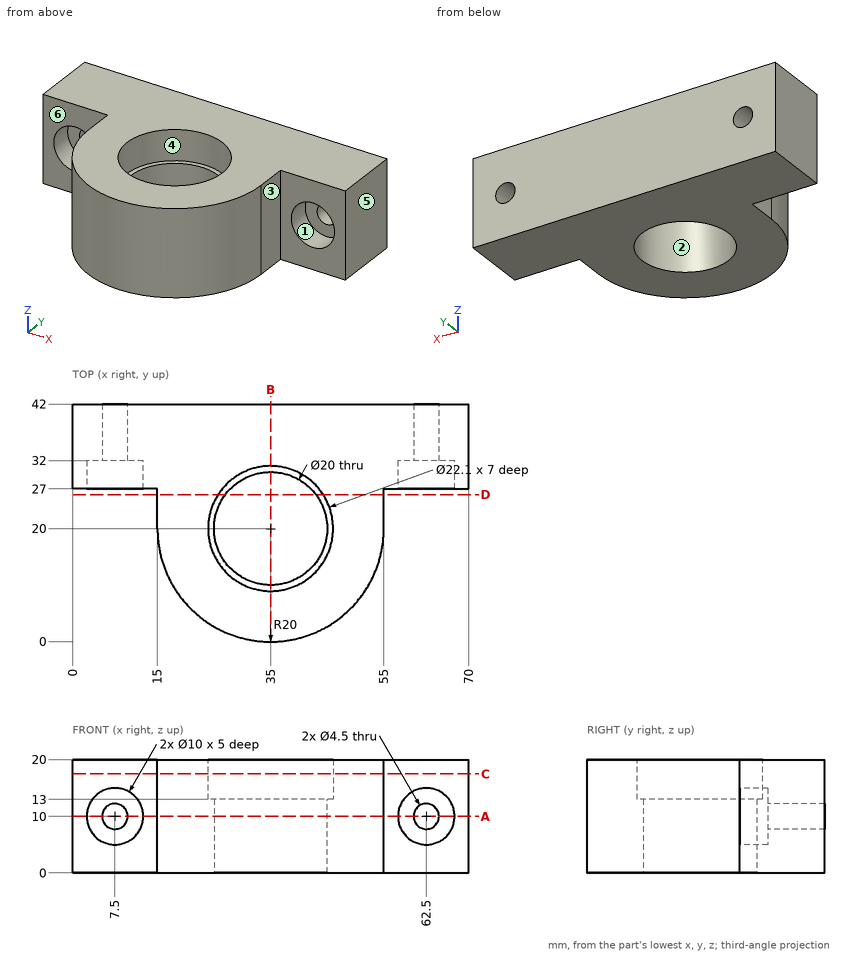
Study the drawing (mm; zero at the part's minimum x, y, z) and answer. A direction names the side the tool comes from. Give positions to 0.01 mm unless a question says otherwise; leave off trailing zeros. Loops run counter-clockwise (first coordinate to the right, second up) from the corner with the lowest first, then second, coordinate; pieces in that order, holes last. Notation, with made-up numbers: (56, 72.25) -> (93, 72.25) arc R28 cw to (93, 95.25) -> close; hole circle Ø2 at (50.5, 55.25). An arc over 180 degrees is marked (long way). Use a Markdown table: item, result. Add a question column.
1) Consider line 1 along Z through (x, y) = (62.5, 37); line 2 along Y through (x, z) = (35, 5.5); line 3 along Z through (x, y) = (62.5, 28.75). Determine where each line is inside the solid, lowest interval first.
2) The part is cut by section D-D, the plane y = 26. Determine the outline of the cut face in (x, z).
3) Which of the six approach directions +Z, -Z, +X, -X, +Y, -Y give full straight-line access (tool end or side, diameter ignored) to the marked faces 1, 2 and 3?
4) The part is cut by section B-B, the plane x = 35. Determine the outline of the cut face in (y, z).
5) The part is cut by section A-A, the plane z = 10. Determine the outline of the cut face in (x, y).
6) The part is cut by section C-C, the plane z = 17.5. Determine the outline of the cut face in (x, y), plus the area to 3 significant figures.
7) Each of these flat-tipped pins is pushed along its axis until it touches: P1, Ø12, axis at x = 61.5, z = 14, coming from the -Y side; P2, Ø4, axis at y = 17.5, z = 13, coming from the -X side; P3, Ø2, axis at y = 22, z = 10, coming from the +X side. Where does it stop, or does it pass through?
8) For a pull along X with two mould halves and no side action, classify the marked faces 4, 5 and 6 as +X half, -X half, draft (parallel to the pull), parting line (faces both ways), or undercut.
Reported:
| question | item | result |
|---|---|---|
| 1 | line 1 | z = 0 to 7.75, 12.25 to 20 |
| 1 | line 2 | y = 0 to 10, 30 to 42 |
| 1 | line 3 | z = 0 to 5, 15 to 20 |
| 2 | outline | (15, 0) -> (27, 0) -> (27, 13) -> (25.72, 13) -> (25.72, 20) -> (15, 20) -> close; (43, 0) -> (55, 0) -> (55, 20) -> (44.28, 20) -> (44.28, 13) -> (43, 13) -> close |
| 3 | face 1 | -Y |
| 3 | face 2 | +Z, -Z |
| 3 | face 3 | +Z, -Z, +X, -Y |
| 4 | outline | (0, 0) -> (10, 0) -> (10, 13) -> (8.95, 13) -> (8.95, 20) -> (0, 20) -> close; (30, 0) -> (42, 0) -> (42, 20) -> (31.05, 20) -> (31.05, 13) -> (30, 13) -> close |
| 5 | outline | (0, 27) -> (2.5, 27) -> (2.5, 32) -> (5.25, 32) -> (5.25, 42) -> (0, 42) -> close; (9.75, 32) -> (12.5, 32) -> (12.5, 27) -> (15, 27) -> (15, 20) arc R20 ccw to (55, 20) -> (55, 27) -> (57.5, 27) -> (57.5, 32) -> (60.25, 32) -> (60.25, 42) -> (9.75, 42) -> close; (64.75, 32) -> (67.5, 32) -> (67.5, 27) -> (70, 27) -> (70, 42) -> (64.75, 42) -> close; hole circle Ø20 at (35, 20) |
| 6 | outline | (0, 27) -> (15, 27) -> (15, 20) arc R20 ccw to (55, 20) -> (55, 27) -> (70, 27) -> (70, 42) -> (0, 42) -> close; hole circle Ø22.1 at (35, 20) |
| 6 | area | 1,570 mm^2 |
| 7 | P1 | stops at y = 27 |
| 7 | P2 | stops at x = 15.01 |
| 7 | P3 | stops at x = 55 |
| 8 | face 4 | undercut |
| 8 | face 5 | +X half |
| 8 | face 6 | draft |
